Can you work these out from the model? Positions are in its coordinate system, mm. Face numbers are marked on the shaded views. A direction names the side the tool comes from. Give positions to 0.01 mm unless a question says otherwise; leave off trailing zeros. Loops run counter-clockwise (first coordinate to the right, second up) from the corner with the lowest first, then second, coordinate; pieces in that order, holes last. Notation, with made-up numbers: M -6,-12 L 4,-12 A21 cw 4,25 Z; hole C -6,7 d3. An arc over 180 degrees is marked long. Answer as a JSON object with one key per item and string values.
Autodesk Inventor part; units mm, degrees
ref_plane "YZ Plane" through (0, 0, 0) normal (1, 0, 0) x (0, 1, 0)
ref_plane "XZ Plane" through (0, 0, 0) normal (0, 1, 0) x (-1, 0, 0)
ref_plane "XY Plane" through (0, 0, 0) normal (0, 0, 1) x (1, 0, 0)
sketch "Sketch1" plane through (0, 0, 0) normal (0, 1, 0) x (-1, 0, 0)
  circle A0 centre (0, 0) radius 3
  dimension "d0" = 6
extrude "Extrusion1" add sketch "Sketch1" along normal blind 39
sketch "Sketch2" plane through (0, 39, 0) normal (0, 1, 0) x (1, 0, 0)
  line L0 (-3.7501, -6.4954) -> (-7.5003, 0)
  line L1 (-7.5003, 0) -> (-3.7501, 6.4954)
  line L2 (-7.5003, 0) -> (0, 0) construction
  line L3 (-3.7501, 6.4954) -> (3.7501, 6.4954)
  line L4 (3.7501, 6.4954) -> (7.5003, 0)
  line L5 (3.7501, -6.4954) -> (7.5003, 0)
  line L6 (3.7501, -6.4954) -> (-3.7501, 6.4954) construction
  line L7 (3.7501, 6.4954) -> (-3.7501, -6.4954) construction
  line L8 (7.5003, 0) -> (-7.5003, 0) construction
  line L9 (3.7501, -6.4954) -> (-3.7501, -6.4954)
  dimension "d13" = 7.5003
  dimension "d18" = 7.5003
  dimension "d19" = 60
  dimension "d20" = 7.5003
  dimension "d21" = 120
  dimension "d22" = 120
extrude "Extrusion2" add sketch "Sketch2" along normal blind 4
thread "Thread2"
chamfer "Chamfer1" distance 1 angle 45 6 edges at (0, 43, 6.4954) (5.6252, 43, 3.2477) (5.6252, 43, -3.2477) (0, 43, -6.4954) (-5.6252, 43, -3.2477) (-5.6252, 43, 3.2477)
equation "\"d13\" = d9"
equation "\"d18\" = d13"
equation "\"d20\" = d9"
properties part number "Bolt" material "Aluminum 6061-AHC"
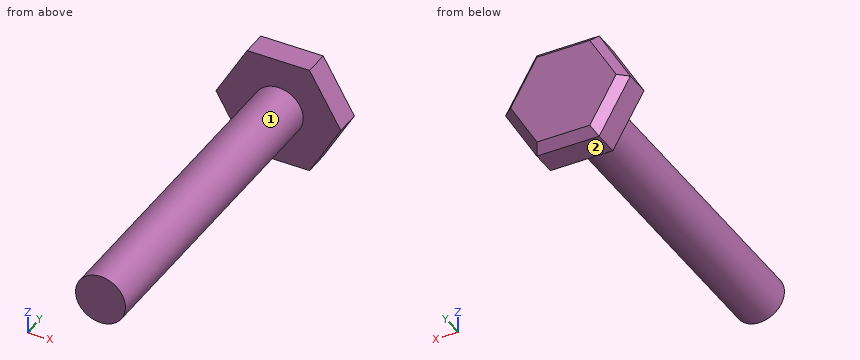
1) Suppose I cut it at D-D, the plane x = 4.25. Write out the boundary of the cut face in (y, z), and give its area (3 significant figures).
Answer list:
{"outline": "M 39,-5.63 L 42,-5.63 L 43,-3.63 L 43,3.63 L 42,5.63 L 39,5.63 Z", "area": "43.0 mm^2"}
2) Will these pins go through, and if not, where does the flat tip stop? pin 1 Ø8 at (x, y) = (4.5, 5) entering from +Z; pin 2 Ø4 at (y, z) = (23, 4.5) entering from -X; pin 3 Ø4 at (y, z) = (27.5, -2.5) entering from +X.
Answer list:
{"pin 1": "z = 2.96", "pin 2": "x = -1.66", "pin 3": "x = 2.96"}
3) Please list where these lines run through material, in increasing order: line 1 along Y through (x, z) = (1.75, 3.5); line 2 along Z through (x, y) = (1.75, 12.5). Write a range as from..to.
Answer list:
{"line 1": "39..43", "line 2": "-2.44..2.44"}
4) Suppose I cut it at B-B, the plane z = -1. Write out the boundary of the cut face in (x, y), and give its area (3 significant figures).
Answer list:
{"outline": "M -6.92,39 L -2.83,39 L -2.83,0 L 2.83,0 L 2.83,39 L 6.92,39 L 6.92,42 L 5.77,43 L -5.77,43 L -6.92,42 Z", "area": "275 mm^2"}
5) Suppose I cut it at A-A, the plane x = 0. Write out the boundary of the cut face in (y, z), and give its area (3 significant figures).
Answer list:
{"outline": "M 0,-3 L 39,-3 L 39,-6.5 L 42,-6.5 L 43,-5.5 L 43,5.5 L 42,6.5 L 39,6.5 L 39,3 L 0,3 Z", "area": "285 mm^2"}
6) Suppose I cut it at C-C, the plane y = 18. Write out the boundary of the cut face in (x, z), and give its area (3 significant figures).
Answer list:
{"outline": "C 0,0 d6", "area": "28.3 mm^2"}
7) For the marked faces 1 and 2, which set-ups out of +Z, -Z, +X, -X, +Y, -Y let a thin tool reach every point of the face, with its end or its side?
Answer list:
{"face 1": "-Y", "face 2": "-Z, +X, -X, +Y, -Y"}
